```python
from build123d import *

# Parameters (mm, degrees)
SKETCH1_W                = 61
SKETCH1_H                = 80
BOSS_EXTRUDE1_DEPTH      = 30
SKETCH2_W                = 54
SKETCH2_H                = 74
CUT_EXTRUDE1_DEPTH       = 27
BOSS_EXTRUDE3_DEPTH      = 80
BOSS_EXTRUDE2_DEPTH      = 4
SKETCH5_R                = 1.6
CUT_EXTRUDE3_DEPTH       = 31
CUT_EXTRUDE4_DEPTH       = 3
CUT_EXTRUDE6_DEPTH       = 81
SKETCH16_R               = 3.1
CUT_EXTRUDE8_DEPTH       = 69.619253581
FILLET1_R                = 5
CUT_EXTRUDE9_START       = -25
SKETCH17_R               = 6.5
CUT_EXTRUDE9_DEPTH       = 10
CUT_EXTRUDE10_START      = -30
CUT_EXTRUDE10_DEPTH      = 20
FILLET2_R                = 20
CUT_EXTRUDE11_REACH      = 82
SKETCH19_R               = 1.6
SKETCH20_W               = 6
SKETCH20_H               = 16
CUT_EXTRUDE12_DEPTH      = 78
CUT_EXTRUDE12_DEPTH_BACK = 4
SKETCH21_W               = 5
SKETCH21_H               = 6
SKETCH21_R               = 1.6
SKETCH21_W_2             = 6
BOSS_EXTRUDE4_DEPTH      = 17
FILLET4_R                = 2
CUT_EXTRUDE13_START      = -77
SKETCH22_R               = 1.6
CUT_EXTRUDE13_DEPTH      = 4


with BuildPart() as part:
    # Sketch1 → Boss-Extrude1 (new body)
    with BuildSketch(Plane(origin=(0, 0, 0), x_dir=(1, 0, 0), z_dir=(0, 1, 0))):
        Rectangle(SKETCH1_W, SKETCH1_H)
    extrude(amount=BOSS_EXTRUDE1_DEPTH)

    # Sketch2 → Cut-Extrude1 (cut)
    with BuildSketch(Plane(origin=(0, 30, 0), x_dir=(1, 0, 0), z_dir=(0, 1, 0))):
        with Locations((0.5, 0)):
            Rectangle(SKETCH2_W, SKETCH2_H)
    extrude(amount=-CUT_EXTRUDE1_DEPTH, mode=Mode.SUBTRACT)

    # Sketch11 → Boss-Extrude3 (add)
    with BuildSketch(Plane.XY.offset(40)):
        Polygon((-30.5, 30), (-40.5, 30), (-58.119022192, 15.215884977), (-58.119022192, 0), (-30.5, 0), align=None)
    extrude(amount=-BOSS_EXTRUDE3_DEPTH)

    # Sketch7 → Boss-Extrude2 (add)
    with BuildSketch(Plane(origin=(0, 3, 0), x_dir=(1, 0, 0), z_dir=(0, 1, 0))):
        Polygon((27.5, -25), (15.5, -37), (27.5, -37), align=None)
        Polygon((27.5, 25), (15.5, 37), (27.5, 37), align=None)
        Polygon((-26.5, 25), (-14.5, 37), (-26.5, 37), align=None)
        Polygon((-14.5, -37), (-26.5, -25), (-26.5, -37), align=None)
    extrude(amount=BOSS_EXTRUDE2_DEPTH)

    # Sketch5 → Cut-Extrude3 (cut, through all)
    with BuildSketch(Plane.XZ):
        with Locations((-24, -34)):
            Circle(SKETCH5_R)
        with Locations((-24, 34)):
            Circle(SKETCH5_R)
        with Locations((26, 34)):
            Circle(SKETCH5_R)
        with Locations((26, -34)):
            Circle(SKETCH5_R)
    extrude(amount=-CUT_EXTRUDE3_DEPTH, mode=Mode.SUBTRACT)

    # Sketch8 → Cut-Extrude4 (cut)
    with BuildSketch(Plane.XZ):
        Polygon((-25.625, 36.814582562), (-27.25, 34), (-25.625, 31.185417438), (-22.375, 31.185417438), (-20.75, 34), (-22.375, 36.814582562), align=None)
        Polygon((24.375, 36.814582562), (22.75, 34), (24.375, 31.185417438), (27.625, 31.185417438), (29.25, 34), (27.625, 36.814582562), align=None)
        Polygon((-25.625, -31.185417438), (-27.25, -34), (-25.625, -36.814582562), (-22.375, -36.814582562), (-20.75, -34), (-22.375, -31.185417438), align=None)
        Polygon((24.375, -31.185417438), (22.75, -34), (24.375, -36.814582562), (27.625, -36.814582562), (29.25, -34), (27.625, -31.185417438), align=None)
    extrude(amount=-CUT_EXTRUDE4_DEPTH, mode=Mode.SUBTRACT)

    # Sketch12 → Cut-Extrude6 (cut, through all)
    with BuildSketch(Plane.XY.offset(40)):
        Polygon((-58.119022192, 15.215884977), (-45.351378719, 0), (-58.119022192, 0), align=None)
    extrude(amount=-CUT_EXTRUDE6_DEPTH, mode=Mode.SUBTRACT)

    # Sketch16 → Cut-Extrude8 (cut, through all)
    with BuildSketch(Plane(origin=(-31.505740697, 37.547079664, 0), x_dir=(0.766044443, 0.64278761, 0), z_dir=(-0.64278761, 0.766044443, 0))):
        with Locations((-23.241171656, 25)):
            Circle(SKETCH16_R)
        with Locations((-23.241171656, -25)):
            Circle(SKETCH16_R)
    extrude(amount=-CUT_EXTRUDE8_DEPTH, mode=Mode.SUBTRACT)

    # Fillet1
    fillet1_edges = [part.edges().sort_by_distance(p)[0] for p in [
        (-26.5, 3, 0),
    ]]
    fillet(fillet1_edges, radius=FILLET1_R)

    # Sketch17 → Cut-Extrude9 (cut)
    with BuildSketch(Plane(origin=(-31.505740697, 37.547079664, 0), x_dir=(0.766044443, 0.64278761, 0), z_dir=(-0.64278761, 0.766044443, 0)).offset(CUT_EXTRUDE9_START)):
        with Locations((-23.241171656, -25)):
            Circle(SKETCH17_R)
        with Locations((-23.241171656, 25)):
            Circle(SKETCH17_R)
    extrude(amount=-CUT_EXTRUDE9_DEPTH, mode=Mode.SUBTRACT)

    # Sketch18 → Cut-Extrude10 (cut)
    with BuildSketch(Plane.XY.offset(40).offset(CUT_EXTRUDE10_START)):
        Polygon((-44.812844495, 26.381093775), (-37.803211847, 22.814854282), (-23.803211847, 22.814854282), (-23.803211847, 12.814854282), (-39.803211847, 12.814854282), (-52.986917817, 19.522231865), align=None)
    extrude(amount=-CUT_EXTRUDE10_DEPTH, mode=Mode.SUBTRACT)

    # Fillet2
    fillet2_edges = [part.edges().sort_by_distance(p)[0] for p in [
        (-37.803211847, 22.814854282, 0),
        (-39.803211847, 12.814854282, 0),
    ]]
    fillet(fillet2_edges, radius=FILLET2_R)

    # Sketch19 → Cut-Extrude11 (cut, up to next)
    with BuildSketch(Plane.XY.offset(40), mode=Mode.PRIVATE) as cut_extrude11_sk1:
        with Locations((-8.416221869, 22)):
            Circle(SKETCH19_R)
    cut_extrude11_tool1 = extrude(cut_extrude11_sk1.sketch, amount=-CUT_EXTRUDE11_REACH, mode=Mode.PRIVATE) & part.part
    add(cut_extrude11_tool1.solids().sort_by_distance((-8.416222, 22, 40))[0], mode=Mode.SUBTRACT)
    # Sketch19 → Cut-Extrude11 (cut, up to next)
    with BuildSketch(Plane.XY.offset(40), mode=Mode.PRIVATE) as cut_extrude11_sk2:
        with Locations((-8.416221869, 7)):
            Circle(SKETCH19_R)
    cut_extrude11_tool2 = extrude(cut_extrude11_sk2.sketch, amount=-CUT_EXTRUDE11_REACH, mode=Mode.PRIVATE) & part.part
    add(cut_extrude11_tool2.solids().sort_by_distance((-8.416222, 7, 40))[0], mode=Mode.SUBTRACT)

    # Sketch20 → Cut-Extrude12 (cut, two sides)
    with BuildSketch(Plane(origin=(0, 0, 37), x_dir=(-1, 0, 0), z_dir=(0, 0, -1))) as cut_extrude12_sk:
        with Locations((18.5, 16)):
            Rectangle(SKETCH20_W, SKETCH20_H)
    extrude(amount=CUT_EXTRUDE12_DEPTH, mode=Mode.SUBTRACT)
    extrude(cut_extrude12_sk.sketch, amount=-CUT_EXTRUDE12_DEPTH_BACK, mode=Mode.SUBTRACT)

    # Sketch21 → Boss-Extrude4 (add)
    with BuildSketch(Plane(origin=(0, 7, 0), x_dir=(1, 0, 0), z_dir=(0, 1, 0))):
        with Locations((-24, -34)):
            Rectangle(SKETCH21_W, SKETCH21_H)
        with Locations((-24, -34)):
            Circle(SKETCH21_R, mode=Mode.SUBTRACT)
        with Locations((-24, 34)):
            Rectangle(SKETCH21_W, SKETCH21_H)
        with Locations((-24, 34)):
            Circle(SKETCH21_R, mode=Mode.SUBTRACT)
        with Locations((26, 34)):
            Rectangle(SKETCH21_W_2, SKETCH21_H)
        with Locations((26, 34)):
            Circle(SKETCH21_R, mode=Mode.SUBTRACT)
        with Locations((26, -34)):
            Rectangle(SKETCH21_W_2, SKETCH21_H)
        with Locations((26, -34)):
            Circle(SKETCH21_R, mode=Mode.SUBTRACT)
    extrude(amount=BOSS_EXTRUDE4_DEPTH)

    # Fillet4
    fillet4_edges = [part.edges().sort_by_distance(p)[0] for p in [
        (-21.5, 15.5, 31),
        (-21.5, 15.5, -31),
        (23, 15.5, -31),
        (23, 15.5, 31),
    ]]
    fillet(fillet4_edges, radius=FILLET4_R)

    # Sketch22 → Cut-Extrude13 (cut, through all)
    with BuildSketch(Plane.XY.offset(40).offset(CUT_EXTRUDE13_START)):
        with Locations((11.583778131, 22)):
            Circle(SKETCH22_R)
        with Locations((11.583778131, 7)):
            Circle(SKETCH22_R)
    extrude(amount=-CUT_EXTRUDE13_DEPTH, mode=Mode.SUBTRACT)


solid = part.part
```
Can you work these out from the model? Positions are in its coordinate system, mm. A direction names the side the tool comes from. Coordinates: 2 decimals unless noted, no trailing zeros. Loops run counter-clockwise (first coordinate to the right, second up) from the corner with the lowest first, then second, coordinate; pieces in that order, holes last. Notation, with made-up numbers: M 56,72.5 L 111,72.5 A28 ccw 111,104.5 Z; hole C 32.5,76.25 d5. An arc over 180 degrees is marked long. Put each result on its own line as item: value. Start each with the question number.
(1) Imagine slicing it at D-D on x = -18. List the corners of the cut face in (y, z) for me.
(2) I need wall thicknesses on probe 1 along Z at (x, y) = (-24, 12); probe 2 along Z at (x, y) = (-12.5, 11); probe 3 along X at (y, z) = (11, 34). Which ranges of each line are inside material? Lowest first, please.
(3) Will these pins go through, and if not, where does the flat tip stop? pin 1 Ø1 at (y, z) = (4.5, -17.5) entering from -X; pin 2 Ø2.5 at (x, z) = (-24, -32.5) entering from +Y; pin 3 Ø0.9 at (y, z) = (17, 38.5) entering from -X.
(4) Which directions (+Z, -Z, +X, -X, +Y, -Y) give clear straight access to the entire face, cutting with the end or side of a thin tool? Please do faces 4 (the face through (-15.5, 16, 38)), 5 (the face through (-25.8, 4.7, -24.8)), 6 (the face through (27.5, 27, 36)), 7 (the face through (-22.6, 3, -32.7)).
(5) Imagine slicing it at C-C on x = 6.5. List the corners of the cut face in (y, z) for me, and give its area (3 significant figures).
(6) Imagine slicing it at A-A on x = 26. Give the number of separate pieces and of enclosed holes in the cut face, and give its area (3 significant figures).
(7) We'd pull the mould along X, two halves only. Please class faces 1 (the face through (-53.102, 19.426, 0.56)), 2 (the face through (28.449, 1.479, 35.388)), 3 (the face through (-30, 22.815, 0)): +X half, -X half, draft (parallel to the pull), parting line (faces both ways), or undercut.
(8) Imagine slicing it at B-B on z = 0. List the corners of the cut face in (x, y) for me.
Worked answers:
1. outline: M 0,-40 L 8,-40 L 8,-37 L 7,-37 L 7,-33.5 L 3,-33.5 L 3,33.5 L 7,33.5 L 7,37 L 8,37 L 8,40 L 0,40 Z; M 24,-40 L 30,-40 L 30,-37 L 24,-37 Z; M 24,37 L 30,37 L 30,40 L 24,40 Z
2. probe 1: z = -40 to -35.6, -32.4 to -31, 31 to 32.4, 35.6 to 40
2. probe 2: z = -40 to -37, 37 to 40
2. probe 3: x = -54.58 to -25.6, -22.4 to -21.5, 23 to 24.4, 27.6 to 30.5
3. pin 1: stops at x = -49.55
3. pin 2: stops at y = 24
3. pin 3: stops at x = -56.53
4. face 4: +Z, -Z
4. face 5: none
4. face 6: +Y
4. face 7: -Y
5. outline: M 0,-40 L 30,-40 L 30,-37 L 3,-37 L 3,37 L 30,37 L 30,40 L 0,40 Z
5. area: 402 mm2
6. separate pieces: 3
6. enclosed holes: 0
6. area: 522 mm2
7. face 1: -X half
7. face 2: undercut
7. face 3: draft
8. outline: M -58.12,15.22 L -45.35,0 L 30.5,0 L 30.5,30 L 27.5,30 L 27.5,3 L -21.5,3 A5 cw -26.5,8 L -26.5,12.81 L -35.01,12.81 A20 cw -44.08,14.99 L -52.99,19.52 Z; M -44.81,26.38 L -42.08,24.99 A20 ccw -33.01,22.81 L -26.5,22.81 L -26.5,30 L -40.5,30 Z
